Could you check a few things on this model? Use its own coordinates, in mm. Round coordinates to 2 decimals unless told otherwise and drop trailing zeros. Write each loop counter-clockwise with the first axis right and the second up, starting at its lowest first coordinate (ties: lowest second). Pieces come first, ordered by that corner, then holes. Notation, with made-up numbers: (-23.75, 7.5) - (-13.75, 7.5) arc R26 ccw to (-13.75, 25.5) - close; hole circle Ø8 at (4, 37). An arc over 180 degrees is marked (long way). Put each result on its own line as item: value.
from build123d import *

# Parameters (mm, degrees)
EXTRUSION1_DEPTH        = 200
ESQUISSE2_R             = 2.8
ENL_V_MAT_EXTRU_1_DEPTH = 201
CONG_1_R                = 0.5
CONG_2_R                = 1


with BuildPart() as part:
    # Esquisse1 → Extrusion1 (new body)
    with BuildSketch(Plane.XY):
        Polygon((-2.8, 11), (-2.8, 9.3), (-8.097918472, 9.3), (-3.297918472, 4.5), (3.297918472, 4.5), (8.097918472, 9.3), (2.8, 9.3), (2.8, 11), (11, 11), (11, 2.8), (9.3, 2.8), (9.3, 8.097918472), (4.5, 3.297918472), (4.5, -3.297918472), (9.3, -8.097918472), (9.3, -2.8), (11, -2.8), (11, -11), (2.8, -11), (2.8, -9.3), (8.097918472, -9.3), (3.297918472, -4.5), (-3.297918472, -4.5), (-8.097918472, -9.3), (-2.8, -9.3), (-2.8, -11), (-11, -11), (-11, -2.8), (-9.3, -2.8), (-9.3, -8.097918472), (-4.5, -3.297918472), (-4.5, 3.297918472), (-9.3, 8.097918472), (-9.3, 2.8), (-11, 2.8), (-11, 11), align=None)
    extrude(amount=EXTRUSION1_DEPTH)

    # Esquisse2 → Enlèv. mat.-Extru.1 (cut, through all)
    with BuildSketch(Plane(origin=(0, 0, 0), x_dir=(-1, 0, 0), z_dir=(0, 0, -1))):
        Circle(ESQUISSE2_R)
    extrude(amount=-ENL_V_MAT_EXTRU_1_DEPTH, mode=Mode.SUBTRACT)

    # Congé1
    cong_1_edges = [part.edges().sort_by_distance(p)[0] for p in [
        (-11, 11, 100),
        (11, 11, 100),
        (11, -11, 100),
        (-11, -11, 100),
    ]]
    fillet(cong_1_edges, radius=CONG_1_R)

    # Congé2
    cong_2_edges = [part.edges().sort_by_distance(p)[0] for p in [
        (-4.5, -3.297918472, 100),
        (-4.5, 3.297918472, 100),
        (-3.297918472, 4.5, 100),
        (3.297918472, 4.5, 100),
        (4.5, 3.297918472, 100),
        (4.5, -3.297918472, 100),
        (3.297918472, -4.5, 100),
        (-3.297918472, -4.5, 100),
    ]]
    fillet(cong_2_edges, radius=CONG_2_R)


solid = part.part
(1) Imagine slicing it at A-A, the plane y = 0. List the corners of the cut face in (x, z) for me.
Values found:
outline: (-4.5, 0) - (-2.8, 0) - (-2.8, 200) - (-4.5, 200) - close; (2.8, 0) - (4.5, 0) - (4.5, 200) - (2.8, 200) - close
(2) Please list where these lines run through material, in increasing order: probe 1 along X at (y, z) = (10.25, 143.5); probe 2 along Y at (x, z) = (0, 44.5); probe 3 along X at (y, z) = (3.5, 166). Write a range as from..to.
Values found:
probe 1: x = -11..-2.8, 2.8..11
probe 2: y = -4.5..-2.8, 2.8..4.5
probe 3: x = -11..-9.3, -4.71..4.71, 9.3..11
(3) I'm going to push flat-ended pins straight in: pin 1 (8 mm diameter, centred on x = 3, y = -1.5, fed in from -Z); pin 2 (4.5 mm diameter, centred on x = 0.5, z = 119.5, fed in from +Y). Where does each tip first touch, or does it pass through?
Values found:
pin 1: stops at z = 0
pin 2: stops at y = 4.5
(4) If we mould it in two halves opening along Y, with no side actions, what happens to faces 1 (the face through (-7, -11, 99)), 2 (the face through (-7, 5.8, 98.6)), 3 (the face through (3, 3, 200))? For each: pulls with the +Y half, pulls with the -Y half, needs draft (parallel to the pull), parting line crosses it, or undercut.
Values found:
face 1: pulls with the -Y half
face 2: undercut
face 3: needs draft
